Print and shaded views of the part. All mm, measured from the part's lowest x, y and z. Round coordinates to 2 decimals unless told otherwise and drop trailing zeros. Order: outer loops, then holes, each group sorted by start corner. A loop starts at its lowest first (then second) coordinate and runs counter-clockwise, first axis right, second up. Notation, with made-up numbers: M 24,-2.75 L 54,-2.75 A25 ccw 54,20.25 Z; hole C 51.25,13.5 d2. An arc over 180 degrees is marked long. Use CSV: the item, a comma, the result in double quotes.
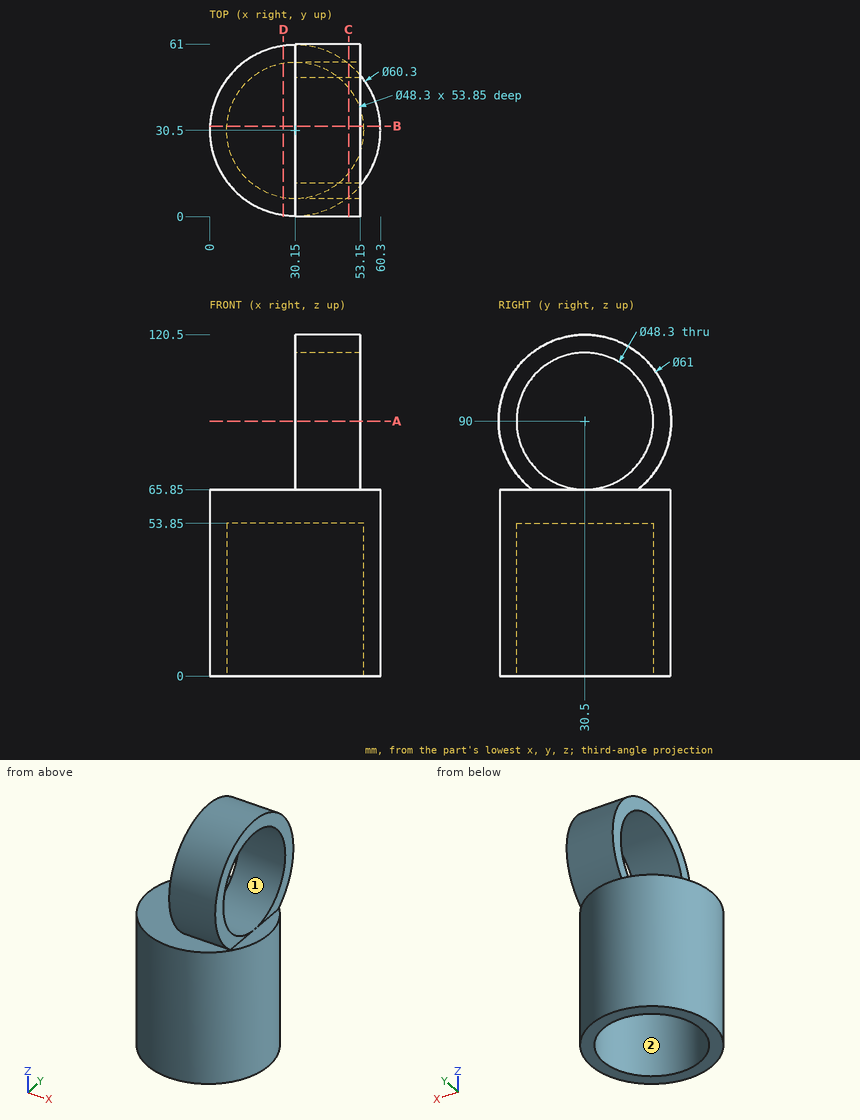
(1) Cut at D-D, the plane x = 26. Give the cut face in (y, z), and give its area (3 significant figures).
Answer block:
outline,"M 0.64,0 L 6.71,0 L 6.71,53.85 L 54.29,53.85 L 54.29,0 L 60.36,0 L 60.36,65.85 L 0.64,65.85 Z"
area,"1,370 mm²"
(2) Wall check: line 1 (Z direction, x = 38.25, y = 30.5); line 2 (Y direction, x = 30.15, z = 37); line 3 (Y direction, x = 44, z = 90). Give the ranges that are in metal, low to high. Write a range as from..to.
Answer block:
line 1,"z = 53.85..65.85, 114.15..120.5"
line 2,"y = 0.35..6.35, 54.65..60.65"
line 3,"y = 0..6.35, 54.65..61"
(3) Cut at A-A, the plane z = 90. Give the cut face in (x, y).
Answer block:
outline,"M 30.15,0 L 53.15,0 L 53.15,6.35 L 30.15,6.35 Z; M 30.15,54.65 L 53.15,54.65 L 53.15,61 L 30.15,61 Z"
(4) Cut at C-C, the plane x = 49. Give the cut face in (y, z).
Answer block:
outline,"M 6.97,0 L 15.4,0 L 15.4,53.85 L 45.6,53.85 L 45.6,0 L 54.03,0 L 54.03,65.85 L 49.13,65.85 A30.5 ccw long 11.87,65.85 L 6.97,65.85 Z; hole C 30.5,90 d48.3"
(5) Two-plate mould, pull along Z, no slides. Class the marked faces 1 and 2: released by +Z, released by -Z, zero draft, split by the parting line, or undercut.
Answer block:
face 1,"undercut"
face 2,"zero draft"
(6) Cut at B-B, the plane y = 32. Give the cut face in (x, z), and give its area (3 significant figures).
Answer block:
outline,"M 0.04,0 L 6.05,0 L 6.05,53.85 L 54.25,53.85 L 54.25,0 L 60.26,0 L 60.26,65.85 L 53.15,65.85 L 53.15,65.9 L 30.15,65.9 L 30.15,65.85 L 0.04,65.85 Z; M 30.15,114.1 L 53.15,114.1 L 53.15,120.46 L 30.15,120.46 Z"
area,"1,520 mm²"
(7) Drop flat-ended pins along their axis: pin 1 (2 mm diameter, centred on x = 26, y = 9, fed in from -Z); pin 2 (4 mm diameter, centred on x = 53, z = 102.5, fed in from +Y); pin 3 (12 mm diameter, centred on y = 54.5, z = 49, fed in from +X). Give the stop position or say it passes through.
Answer block:
pin 1,"stops at z = 53.85"
pin 2,"stops at y = 59.14"
pin 3,"stops at x = 54.34"
